from build123d import *

# Parameters (mm, degrees)
BOX003_W          = 48
BOX003_H          = 78
BOX003_DEPTH      = 2
BOX002_W          = 48
BOX002_H          = 78
BOX002_DEPTH      = 2
CYLINDER006_R     = 41.5
CYLINDER006_DEPTH = 2
CYLINDER005_R     = 42
CYLINDER005_DEPTH = 2
CYLINDER004_R     = 40.5
CYLINDER004_DEPTH = 2
CYLINDER003_R     = 4
CYLINDER003_DEPTH = 26
BOX001_W          = 46
BOX001_H          = 99
BOX001_DEPTH      = 138
BOX_W             = 46
BOX_H             = 99
BOX_DEPTH         = 138
CYLINDER002_R     = 38
CYLINDER002_DEPTH = 138
CYLINDER001_R     = 19.5
CYLINDER001_DEPTH = 15
CYLINDER_R        = 42
CYLINDER_DEPTH    = 154


with BuildPart() as cubo003:
    # Box003 → Box003 (new body)
    with BuildSketch(Plane(origin=(37, -24, -2), x_dir=(0, 1, 0), z_dir=(0, 0, 1))):
        with Locations((24, 39)):
            Rectangle(BOX003_W, BOX003_H)
    extrude(amount=BOX003_DEPTH)


with BuildPart() as cubo002:
    # Box002 → Box002 (new body)
    with BuildSketch(Plane(origin=(-24, -39, -2), x_dir=(1, 0, 0), z_dir=(0, 0, 1))):
        with Locations((24, 39)):
            Rectangle(BOX002_W, BOX002_H)
    extrude(amount=BOX002_DEPTH)


with BuildPart() as base002:
    # Cylinder006 → Cylinder006 (new body)
    with BuildSketch(Plane.XY.offset(-2)):
        Circle(CYLINDER006_R)
    extrude(amount=CYLINDER006_DEPTH)


with BuildPart() as cut006:
    # Cylinder005 → Cylinder005 (new body)
    with BuildSketch(Plane.XY.offset(-2)):
        Circle(CYLINDER005_R)
    extrude(amount=CYLINDER005_DEPTH)

    # Cut006: cut Base002
    add(base002.part, mode=Mode.SUBTRACT)


with BuildPart() as agujero_inferior001:
    # Cylinder004 → Cylinder004 (new body)
    with BuildSketch(Plane.XY.offset(-2)):
        Circle(CYLINDER004_R)
    extrude(amount=CYLINDER004_DEPTH)


with BuildPart() as agujero_cables:
    # Cylinder003 → Cylinder003 (new body)
    with BuildSketch(Plane(origin=(0, -29, 131), x_dir=(1, 0, 0), z_dir=(0, 0, 1))):
        Circle(CYLINDER003_R)
    extrude(amount=CYLINDER003_DEPTH)


with BuildPart() as cubo001:
    # Box001 → Box001 (new body)
    with BuildSketch(Plane(origin=(44, -23, -2), x_dir=(0, 1, 0), z_dir=(0, 0, 1))):
        with Locations((23, 49.5)):
            Rectangle(BOX001_W, BOX001_H)
    extrude(amount=BOX001_DEPTH)


with BuildPart() as cubo:
    # Box → Box (new body)
    with BuildSketch(Plane(origin=(-23, -50, -2), x_dir=(1, 0, 0), z_dir=(0, 0, 1))):
        with Locations((23, 49.5)):
            Rectangle(BOX_W, BOX_H)
    extrude(amount=BOX_DEPTH)


with BuildPart() as agujero_inferior:
    # Cylinder002 → Cylinder002 (new body)
    with BuildSketch(Plane.XY.offset(-2)):
        Circle(CYLINDER002_R)
    extrude(amount=CYLINDER002_DEPTH)


with BuildPart() as agujero_superior:
    # Cylinder001 → Cylinder001 (new body)
    with BuildSketch(Plane.XY.offset(138)):
        Circle(CYLINDER001_R)
    extrude(amount=CYLINDER001_DEPTH)


with BuildPart() as cut009:
    # Cylinder → Cylinder (new body)
    with BuildSketch(Plane.XY.offset(-2)):
        Circle(CYLINDER_R)
    extrude(amount=CYLINDER_DEPTH)

    # Cut: cut Agujero superior
    add(agujero_superior.part, mode=Mode.SUBTRACT)

    # Cut001: cut Agujero inferior
    add(agujero_inferior.part, mode=Mode.SUBTRACT)

    # Cut002: cut Cubo
    add(cubo.part, mode=Mode.SUBTRACT)

    # Cut003: cut Cubo001
    add(cubo001.part, mode=Mode.SUBTRACT)

    # Cut004: cut Agujero cables
    add(agujero_cables.part, mode=Mode.SUBTRACT)

    # Cut005: cut Agujero inferior001
    add(agujero_inferior001.part, mode=Mode.SUBTRACT)

    # Cut007: cut Cut006
    add(cut006.part, mode=Mode.SUBTRACT)

    # Cut008: cut Cubo002
    add(cubo002.part, mode=Mode.SUBTRACT)

    # Cut009: cut Cubo003
    add(cubo003.part, mode=Mode.SUBTRACT)


solid = cut009.part
Geometry: final body of the model. Coordinates: model frame, mm. A direction names the side the tool comes from. Give positions to 0.01 mm unless a question says otherwise; leave off trailing zeros. Write each loop counter-clockwise with the first axis right and the second up, starting at its lowest first coordinate (ties: lowest second). Pieces come first, ordered by that corner, then holes.
(1) Cut plane D-D, the plane x = 14. Return loops of the section in (y, z), then the cut area to 3 significant figures.
(2) Mould query, pull axis X, two halves, no side actions, for faces 4 (the flat face through (-33, -23, 67)), 5 (the cylindrical face through (-29.28, 29.41, -1.01)), 6 (the flat face through (-23, -33, 67)), 7 (the cylindrical face through (29.28, -29.41, -1.01)). Classes: released by +X, released by -X, zero draft, split by the parting line, or undercut.
(3) Access query for faces 1 (the flat face through (33, 23, 67)), 2 (the flat face through (-23, 33, 67)), 3 (the cylindrical face through (26.92, 26.82, 67.05)). Directions: +Z, -Z, +X, -X, +Y, -Y. A direction counts if a zero-diameter tool reaches every point of the face in a straight line with its end or side. Return the directions, or none.
(4) First-contact query: P1, Ø0.6, axis at x = -33.5, z = -1.5, coming from the -Y side; P2, Ø8, axis at y = -30.5, z = 90.5, coming from the +X side; P3, Ø1.5, axis at x = -32, z = 86, coming from the -Y side; P4, Ø12, axis at x = -12, z = 16.5, coming from the +Y side. Flat tips, straight axial feed; report the tip coordinate or a pass-through.
(5) Cut plane B-B, the plane z = 70.5. Return loops of the section in (x, y), then the cut area to 3 significant figures.
(6) Cut plane C-C, the plane y = 0. Return loops of the section in (x, z).
(7) Ray query, line 1 (Y direction, x = 0, z = 144.75); line 2 (X direction, y = 0, z = 147); line 3 (Z direction, x = 38, y = 4). Return the intervals inside material, ascending.
(8) Cut plane A-A, the plane x = 0. Return loops of the section in (y, z), then the cut area to 3 significant figures.
Values follow:
1. outline: (-39.6, 136) - (39.6, 136) - (39.6, 152) - (13.57, 152) - (13.57, 138) - (-13.57, 138) - (-13.57, 152) - (-39.6, 152) - close
1. area: 887 mm2
2. face 4: zero draft
2. face 5: released by -X
2. face 6: undercut
2. face 7: released by +X
3. face 1: -Z, +X, -X
3. face 2: -Z, +Y, -Y
3. face 3: -Z
4. P1: stops at y = -24.9
4. P2: stops at x = 32.58
4. P3: stops at y = -28.06
4. P4: passes through
5. outline: (-35.14, -23) arc R42 ccw to (-23, -35.14) - (-23, -30.25) arc R38 cw to (-30.25, -23) - close; (-35.14, 23) - (-30.25, 23) arc R38 cw to (-23, 30.25) - (-23, 35.14) arc R42 ccw to start; (23, -35.14) arc R42 ccw to (35.14, -23) - (30.25, -23) arc R38 cw to (23, -30.25) - close; (23, 30.25) arc R38 cw to (30.25, 23) - (35.14, 23) arc R42 ccw to (23, 35.14) - close
5. area: 221 mm2
6. outline: (-42, 136) - (42, 136) - (42, 152) - (19.5, 152) - (19.5, 138) - (-19.5, 138) - (-19.5, 152) - (-42, 152) - close
7. line 1: y = -42 to -33, -25 to -19.5, 19.5 to 42
7. line 2: x = -42 to -19.5, 19.5 to 42
7. line 3: z = 136 to 152
8. outline: (-42, 136) - (-33, 136) - (-33, 152) - (-42, 152) - close; (-25, 136) - (42, 136) - (42, 152) - (19.5, 152) - (19.5, 138) - (-19.5, 138) - (-19.5, 152) - (-25, 152) - close
8. area: 670 mm2
